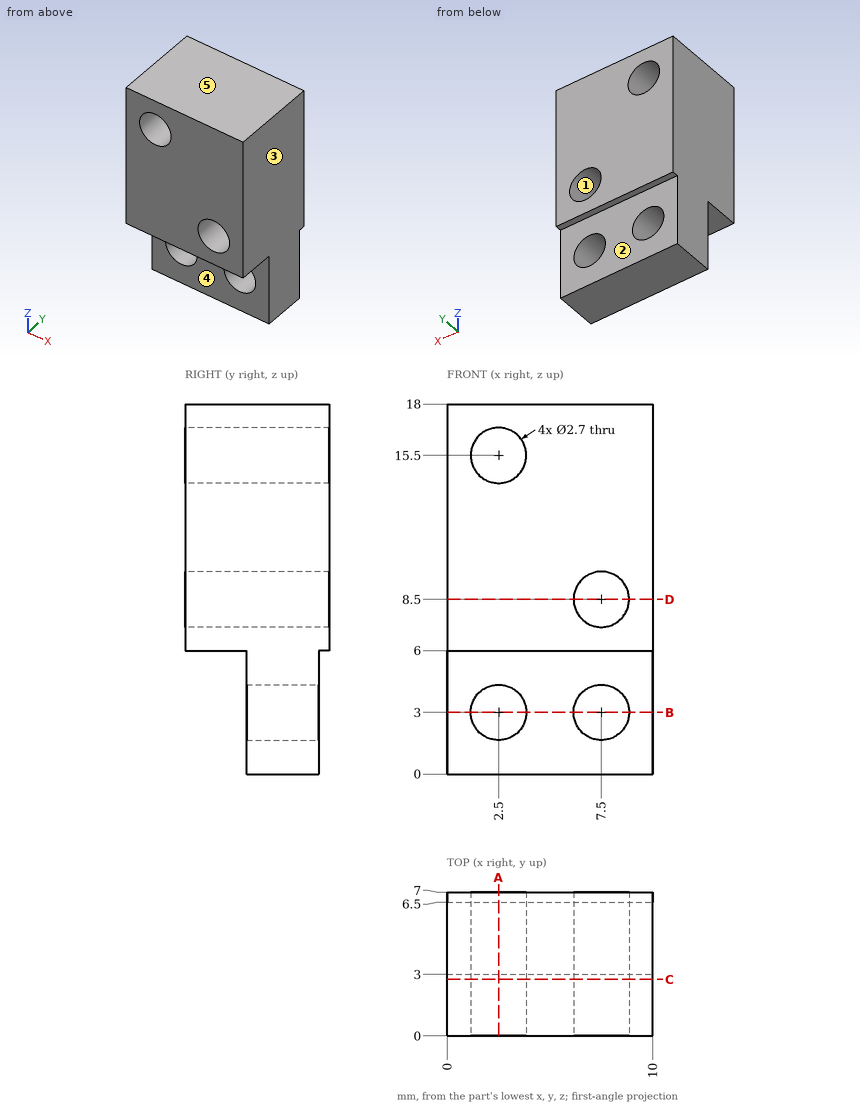
Study the drawing (mm; zero at the part's minimum x, y, z) and answer. A direction names the side the tool comes from. Give positions to 0.01 mm unless a question says otherwise; leave off trailing zeros. Write each loop counter-clockwise with the first axis right and the second up, starting at its lowest first coordinate (ties: lowest second). Pieces come first, ordered by that corner, then holes. Notation, with made-up numbers: (46.25, 11.25) -> (62.25, 11.25) arc R14 cw to (62.25, 35.25) -> close; hole circle Ø5 at (0.25, 23). An arc over 180 degrees is marked (long way). Answer in a Markdown table with one row per item.
1) A tool of negligible diameter and unlimited length cuts with its end or side. For the marked faces 4 and 5, from which of +Z, -Z, +X, -X, +Y, -Y can it reach the whole face along a straight path? Write none if from no direction.
Results list:
| item | result |
|---|---|
| face 4 | -Z, +X, -X, -Y |
| face 5 | +Z, +X, -X, +Y, -Y |
2) Each of these flat-tipped pins is pushed along its axis until it touches: pin 1 Ø5 at (x, z) = (3, 2) entering from -Y; pin 2 Ø1.8 at (x, z) = (5, 4) entering from +Y; pin 3 Ø3.5 at (x, y) = (3, 1) entering from -Z. Where does it stop, or does it pass through?
Results list:
| item | result |
|---|---|
| pin 1 | y = 3 |
| pin 2 | y = 6.5 |
| pin 3 | z = 6 |
3) Section A-A on x = 2.5 is taken. Give the vertices of the cut face in (y, z).
Results list:
| item | result |
|---|---|
| outline | (0, 6) -> (3, 6) -> (3, 4.35) -> (6.5, 4.35) -> (6.5, 6) -> (7, 6) -> (7, 14.15) -> (0, 14.15) -> close; (0, 16.85) -> (7, 16.85) -> (7, 18) -> (0, 18) -> close; (3, 0) -> (6.5, 0) -> (6.5, 1.65) -> (3, 1.65) -> close |
4) Section D-D on z = 8.5 is taken. Give the vertices of the cut face in (x, y).
Results list:
| item | result |
|---|---|
| outline | (0, 0) -> (6.15, 0) -> (6.15, 7) -> (0, 7) -> close; (8.85, 0) -> (10, 0) -> (10, 7) -> (8.85, 7) -> close |
5) Determine the mould class of the marked faces 1, 2 and 3 for opening direction X: released by +X, released by -X, zero draft, split by the parting line, or undercut.
Results list:
| item | result |
|---|---|
| face 1 | undercut |
| face 2 | zero draft |
| face 3 | released by +X |
6) Section B-B on z = 3 is taken. Give the vertices of the cut face in (x, y), plus the area to 3 significant figures.
Results list:
| item | result |
|---|---|
| outline | (0, 3) -> (1.15, 3) -> (1.15, 6.5) -> (0, 6.5) -> close; (3.85, 3) -> (6.15, 3) -> (6.15, 6.5) -> (3.85, 6.5) -> close; (8.85, 3) -> (10, 3) -> (10, 6.5) -> (8.85, 6.5) -> close |
| area | 16.1 mm^2 |
7) Straight lines are drawn through the part: line 1 (Z direction, x = 7.5, y = 4.5); line 2 (Z direction, x = 2.5, y = 5); line 3 (X direction, y = 5.75, z = 8.5). For each, find the intervals that lie inside material, in ascending order. Write a range as [from, to].
Results list:
| item | result |
|---|---|
| line 1 | [0, 1.65], [4.35, 7.15], [9.85, 18] |
| line 2 | [0, 1.65], [4.35, 14.15], [16.85, 18] |
| line 3 | [0, 6.15], [8.85, 10] |
8) Section C-C on y = 2.75 is taken. Give the vertices of the cut face in (x, z).
Results list:
| item | result |
|---|---|
| outline | (0, 6) -> (10, 6) -> (10, 18) -> (0, 18) -> close; hole circle Ø2.7 at (2.5, 15.5); hole circle Ø2.7 at (7.5, 8.5) |
